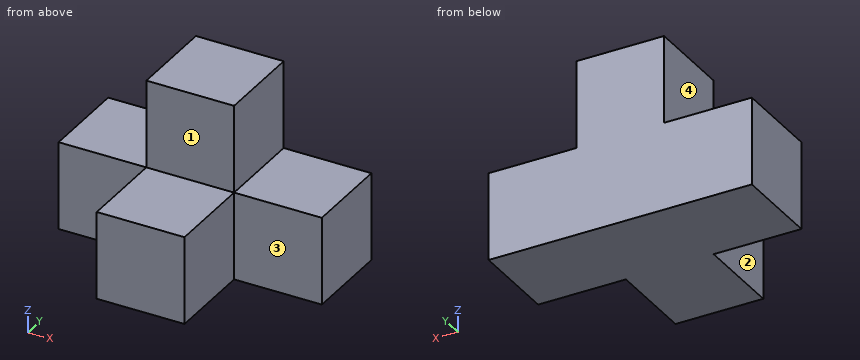
from build123d import *

# Parameters (mm, degrees)
F0_W     = 25.4
F0_H     = 25.4
F1_DEPTH = 50.8
F2_DEPTH = 25.4


with BuildPart() as f1:
    # F0 (on Front) → F1 (new body)
    with BuildSketch(Plane.XZ):
        with Locations((-2.776934, -7.56451)):
            Rectangle(F0_W, F0_H)
    extrude(amount=F1_DEPTH)

    # F0 (on Front) → F2 (join)
    with BuildSketch(Plane.XZ):
        with Locations((-28.176934, -7.56451)):
            Rectangle(F0_W, F0_H)
        with Locations((-2.776934, 17.83549)):
            Rectangle(F0_W, F0_H)
        with Locations((22.623066, -7.56451)):
            Rectangle(F0_W, F0_H)
    extrude(amount=F2_DEPTH)


solid = f1.part
Here's how the part is built. I have some questions about the finished solid (model axes, mm). Face numbers are marked on the shaded views. A direction names the side the tool comes from. Coordinates: 2 decimals unless noted, no trailing zeros. Loops run counter-clockwise (first coordinate to the right, second up) from the corner with the lowest first, then second, coordinate; pieces in that order, holes last.
1. I need wall thicknesses on L1, parallel to X at y = -12.5, z = 6.5; L2, parallel to Z at x = -28, y = -3.5; L3, parallel to Y at x = 24.5, z = 0. Which ranges of each line are inside material? Lowest first, please.
2. For the marked faces 1, 2, 3 and 4, which set-ups out of +Z, -Z, +X, -X, +Y, -Y let a thin tool reach every point of the face, with its end or its side?
3. Imagine slicing it at D-D, the plane y = -36.5. Please give me the cut outline in (x, z), and give its area (3 significant figures).
4. Imagine slicing it at B-B, the plane y = -5. Please give me the cut outline in (x, z).
5. Imagine slicing it at C-C, the plane x = -10.5. Please give me the cut outline in (y, z), and give its area (3 significant figures).
6. For P1, Ø12.5, axis at y = -37, z = -13.5, coming from the +X side; P2, Ø12.5, axis at x = -22, y = -13.5, coming from the +Z side; P3, Ø20.5, axis at x = -8, z = 19.5, coming from the -Y side, each with a flat end and sliding along its axis, tell me the tip position at first contact or that it passes through.
7. Imagine slicing it at A-A, the plane z = -3. Please give me the cut outline in (x, y), and give its area (3 significant figures).
Taken from the geometry:
1. L1: x = -15.48 to 9.92
1. L2: z = -20.26 to 5.14
1. L3: y = -25.4 to 0
2. face 1: +Z, +X, -X, -Y
2. face 2: +Z, -Z, -X, -Y
2. face 3: +Z, -Z, +X, -Y
2. face 4: +Z, -X, +Y, -Y
3. outline: (-15.48, -20.26) - (9.92, -20.26) - (9.92, 5.14) - (-15.48, 5.14) - close
3. area: 645 mm2
4. outline: (-40.88, -20.26) - (35.32, -20.26) - (35.32, 5.14) - (9.92, 5.14) - (9.92, 30.54) - (-15.48, 30.54) - (-15.48, 5.14) - (-40.88, 5.14) - close
5. outline: (-50.8, -20.26) - (0, -20.26) - (0, 30.54) - (-25.4, 30.54) - (-25.4, 5.14) - (-50.8, 5.14) - close
5. area: 1,940 mm2
6. P1: stops at x = 9.92
6. P2: stops at z = 5.14
6. P3: stops at y = -25.4
7. outline: (-40.88, -25.4) - (-15.48, -25.4) - (-15.48, -50.8) - (9.92, -50.8) - (9.92, -25.4) - (35.32, -25.4) - (35.32, 0) - (-40.88, 0) - close
7. area: 2,580 mm2
